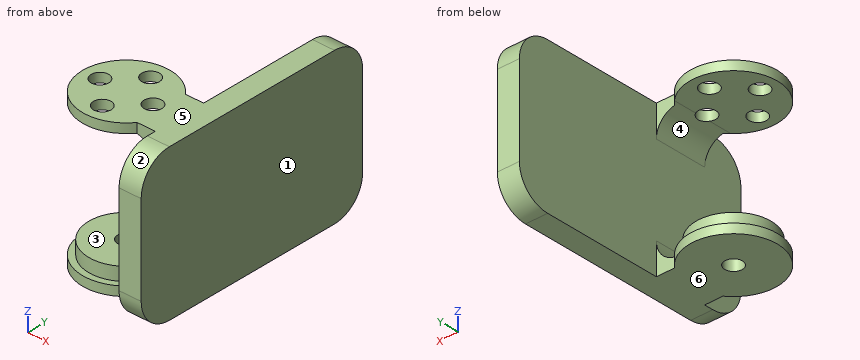
from build123d import *

# Parameters (mm, degrees)
F1_DEPTH      = 17.15
F3_DEPTH      = 40.001
F3_DEPTH_BACK = 15.001
F5_R          = 8.5
F6_DEPTH      = 3
F7_R          = 2
F8_DEPTH      = 5.1010001
F9_R          = 2
F10_DEPTH     = 17.15
F11_R         = 7


with BuildPart() as f1:
    # F0 (on Top) → F1 (new body)
    with BuildSketch(Plane.XY):
        with BuildLine():
            Line((12, 6), (7.874642849, 6))
            ThreePointArc((7.874642849, 6), (-9.9, 0), (7.874642849, -6))
            Line((7.874642849, -6), (12, -6))
            Line((12, -6), (12, -15))
            Line((12, -15), (17, -15))
            Line((17, -15), (17, 40))
            Line((17, 40), (12, 40))
            Line((12, 40), (12, 6))
        make_face()
    extrude(amount=F1_DEPTH)

    # F2 (on Front) → F3 (cut, two sides)
    with BuildSketch(Plane.XZ) as f3_sk:
        with BuildLine():
            Line((7, 15.05), (-20, 15.05))
            Line((-20, 15.05), (-20, 0))
            Line((-20, 0), (12, 0))
            Line((12, 0), (12, 10.05))
            ThreePointArc((12, 10.05), (10.5355339059, 13.5855339059), (7, 15.05))
        make_face()
    extrude(amount=-F3_DEPTH, mode=Mode.SUBTRACT)
    extrude(f3_sk.sketch, amount=F3_DEPTH_BACK, mode=Mode.SUBTRACT)

    # F4: F1 across plane


with BuildPart() as f1_1:
    add(f1.part)
    add(f1.part.mirror(Plane.XY))

    # F5 (on face) → F6 (join)
    with BuildSketch(Plane.XY.offset(-15.05)):
        Circle(F5_R)
    extrude(amount=F6_DEPTH)

    # F7 (on face) → F8 (cut, through all)
    with BuildSketch(Plane.XY.offset(-12.05)):
        Circle(F7_R)
    extrude(amount=-F8_DEPTH, mode=Mode.SUBTRACT)

    # F9 (on face) → F10 (cut, through all)
    with BuildSketch(Plane.XY.offset(17.15)):
        with Locations((6, 0)):
            Circle(F9_R)
        with Locations((0, -6)):
            Circle(F9_R)
        with Locations((-6, 0)):
            Circle(F9_R)
        with Locations((0, 6)):
            Circle(F9_R)
    extrude(amount=-F10_DEPTH, mode=Mode.SUBTRACT)

    # F11
    f11_edges = [f1_1.edges().sort_by_distance(p)[0] for p in [
        (14.5, 40, 17.15),
        (14.5, 40, -17.15),
        (14.5, -15, -17.15),
        (14.5, -15, 17.15),
    ]]
    fillet(f11_edges, radius=F11_R)


solid = f1_1.part
Check sheet for the modelled part. Datum: model origin and axes. Units: mm. Face numbers are marked on the shaded views. A direction names the side the tool comes from. Give positions to 0.01 mm unless a question says otherwise; leave off trailing zeros. Loops run counter-clockwise (first coordinate to the right, second up) from the corner with the lowest first, then second, coordinate; pieces in that order, holes last. Notation, with made-up numbers: M -31.75,50.25 L 24.25,50.25 A7 ccw 24.25,57.25 Z; hole C -34,-10 d3. An arc over 180 degrees is marked long. Answer as a JSON object with one key per item and string values. Group by question number.
Q1. Cross-section at A-A on x = 0. Record the cut outline in (y, z), then the cut area to 3 significant figures.
Q2. Material ranges on line 1 along Y through (x, z) = (0, 16); line 2 along Y through (x, z) = (0, -14.4); line 3 along X through (y, z) = (27.5, 2.5), recorded low to high. Write a range as [from, to].
Q3. Cross-section at D-D on z = 11. Record the cut outline in (x, y).
Q4. Release check for a two-part mould opening along Z. For the marked faces 4, 5 and 6 record: released by +Z, released by -Z, zero draft, split by the parting line, or undercut.
Q5. Cross-section at B-B on x = -6. Record the cut outline in (y, z).
Q6. Access from +Z, -Z, +X, -X, +Y, -Y to the whole of each face (thin tool, end or side, straight path). Record for the marked faces 1, 2 and 3.
Q7. Cross-section at C-C on y = 0. Record the cut outline in (x, z), then the cut area to 3 significant figures.
Q8. Go/stop test with flat-tipped pins: P1, Ø4.5, axis at x = 10.5, z = -15, coming from the +Y side; P2, Ø12, axis at x = 3.5, z = -13, coming from the +Y side; P3, Ø3.5, axis at x = -6, y = 0, coming from the +Z side; P4, Ø2, axis at x = 9, z = 12, coming from the +Y side. Record where each tip stops, or that it passes through.
Evaluation:
{
 "1": {"outline": "M -9.9,-17.15 L -2,-17.15 L -2,-12.05 L -8.5,-12.05 L -8.5,-15.05 L -9.9,-15.05 Z; M -9.9,15.05 L -8,15.05 L -8,17.15 L -9.9,17.15 Z; M -4,15.05 L 4,15.05 L 4,17.15 L -4,17.15 Z; M 2,-17.15 L 9.9,-17.15 L 9.9,-15.05 L 8.5,-15.05 L 8.5,-12.05 L 2,-12.05 Z; M 8,15.05 L 9.9,15.05 L 9.9,17.15 L 8,17.15 Z", "area": "97.0 mm2"},
 "2": {"line 1": "y = [-9.9, -8], [-4, 4], [8, 9.9]", "line 2": "y = [-8.5, -2], [2, 8.5]", "line 3": "x = [12, 17]"},
 "3": {"outline": "M 11.91,-6 L 12,-6 L 12,-14.95 L 17,-14.95 L 17,39.95 L 12,39.95 L 12,6 L 11.91,6 Z"},
 "4": {"face 4": "undercut", "face 5": "released by +Z", "face 6": "released by -Z"},
 "5": {"outline": "M -7.87,-17.15 L 7.87,-17.15 L 7.87,-15.05 L 6.02,-15.05 L 6.02,-12.05 L -6.02,-12.05 L -6.02,-15.05 L -7.87,-15.05 Z; M -7.87,15.05 L -2,15.05 L -2,17.15 L -7.87,17.15 Z; M 2,15.05 L 7.87,15.05 L 7.87,17.15 L 2,17.15 Z"},
 "6": {"face 1": "+Z, -Z, +X, +Y, -Y", "face 2": "+Z, +X, -Y", "face 3": "-X, +Y, -Y"},
 "7": {"outline": "M -9.9,-17.15 L -2,-17.15 L -2,-12.05 L -8.5,-12.05 L -8.5,-15.05 L -9.9,-15.05 Z; M -9.9,15.05 L -8,15.05 L -8,17.15 L -9.9,17.15 Z; M -4,15.05 L 4,15.05 L 4,17.15 L -4,17.15 Z; M 2,-17.15 L 17,-17.15 L 17,17.15 L 8,17.15 L 8,14.95 A5 cw 12,10.05 L 12,-10.05 A5 cw 8.5,-14.82 L 8.5,-12.05 L 2,-12.05 Z", "area": "288 mm2"},
 "8": {"P1": "stops at y = 39.24", "P2": "stops at y = 9.9", "P3": "stops at z = -12.05", "P4": "passes through"}
}
